CAD build for the part. Positions are in the model's coordinates, mm. A direction names the side the tool comes from. Coordinates: 2 decimals unless noted, no trailing zeros. Order: outer loops, then holes, each group sorted by start corner. A loop starts at its lowest first (then second) coordinate and runs counter-clockwise, first axis right, second up. Notation, with made-up numbers: (-14.75, 54.25) - (9.25, 54.25) arc R16 ccw to (9.25, 83.25) - close; hole circle Ø8 at (82, 89.5). An arc over 180 degrees is marked (long way). Return JSON: item names as keys, results as strings.
from build123d import *

# Parameters (mm, degrees)
EXTRUDE_1_DEPTH                 = 220
SKETCH_3_W                      = 130
SKETCH_3_H                      = 90
CUT_EXTRUDE_1_DEPTH             = 585.29444632
EXTRUDE_5_DEPTH                 = 10
EXTRUDE_START                   = -130
EXTRUDE_6_DEPTH                 = 260
EXTRUDE_START_2                 = -220
EXTRUDE_6_2_DEPTH               = 125
EXTRUDE_START_3                 = 95
EXTRUDE_6_3_DEPTH               = 125
EXTRUDE_START_4                 = -76.923226389
EXTRUDE_6_4_DEPTH               = 136.923226389
CUT_EXTRUDE_2_DEPTH             = 585.29444632
SKETCH_13_W                     = 90
SKETCH_13_H                     = 60
EXTRUDE_7_DEPTH                 = 10
EXTRUDE_10_REACH                = 649.534
SKETCH_16_W                     = 90
SKETCH_16_H                     = 60
EXTRUDE_10_DIRECTION_2_REACH    = 649.534
SKETCH_17_W                     = 65
SKETCH_17_H                     = 190
SKETCH_17_W_2                   = 95
EXTRUDE_15_DEPTH                = 5
CUT_EXTRUDE_3_REACH             = 649.534
CUT_EXTRUDE_3_DIRECTION_2_REACH = 649.534


with BuildPart() as part:
    # Эскиз1 → Бобышка-Вытянуть1 (new, symmetric)
    with BuildSketch(Plane.XY):
        Polygon((-219.125113365, -100), (219.125113365, -100), (530, -45.184369862), (530, -55.33863598), (220, -110), (-220, -110), (-530, -55.33863598), (-530, -45.184369862), align=None)
    extrude(amount=EXTRUDE_1_DEPTH, both=True)

    # Эскиз3 → Вырез-Вытянуть1 (cut, through all)
    with BuildSketch(Plane(origin=(0, 0, 0), x_dir=(1, 0, 0), z_dir=(0, 1, 0))):
        with Locations((-465, 175)):
            Rectangle(SKETCH_3_W, SKETCH_3_H)
        with Locations((465, 175)):
            Rectangle(SKETCH_3_W, SKETCH_3_H)
        with Locations((465, -175)):
            Rectangle(SKETCH_3_W, SKETCH_3_H)
        with Locations((-465, -175)):
            Rectangle(SKETCH_3_W, SKETCH_3_H)
    extrude(amount=-CUT_EXTRUDE_1_DEPTH, mode=Mode.SUBTRACT)

    # Эскиз9 → Бобышка-Вытянуть5 (add)
    with BuildSketch(Plane.XY.offset(130)):
        Polygon((-530, -45.184369862), (-400, -68.106877354), (-400, 60), (-530, 60), align=None)
        Polygon((400, -68.106877354), (400, 60), (530, 60), (530, -45.184369862), align=None)
    extrude_5 = extrude(amount=-EXTRUDE_5_DEPTH)

    # Зеркальное отражение3: Бобышка-Вытянуть5 across plane
    add(extrude_5.mirror(Plane.XY))

    # Бобышка-Вытянуть6: read off the stored shape, not the designer's step
    # Бобышка-Вытянуть6 outline → Бобышка-Вытянуть6 (add)
    with BuildSketch(Plane.XY.offset(EXTRUDE_START)):
        Polygon((-530, 60), (-530, -45.184369862), (-520, -46.947639669), (-520, 60), align=None)
        Polygon((530, -45.184369862), (530, 60), (520, 60), (520, -46.947639669), align=None)
    extrude(amount=EXTRUDE_6_DEPTH)

    # Extrude 6 2 outline → Extrude 6 2 (add)
    with BuildSketch(Plane.XY.offset(EXTRUDE_START_2)):
        Polygon((-350, 60), (-350, -76.923226389), (-340, -78.686496196), (-340, 60), align=None)
        Polygon((350, -76.923226389), (350, 60), (340, 60), (340, -78.686496196), align=None)
    extrude(amount=EXTRUDE_6_2_DEPTH)

    # Extrude 6 3 outline → Extrude 6 3 (add)
    with BuildSketch(Plane.XY.offset(EXTRUDE_START_3)):
        Polygon((-350, 60), (-350, -76.923226389), (-340, -78.686496196), (-340, 60), align=None)
        Polygon((350, -76.923226389), (350, 60), (340, 60), (340, -78.686496196), align=None)
    extrude(amount=EXTRUDE_6_3_DEPTH)

    # Extrude 6 4 outline → Extrude 6 4 (add)
    with BuildSketch(Plane(origin=(0, 0, 0), x_dir=(1, 0, 0), z_dir=(0, 1, 0)).offset(EXTRUDE_START_4)):
        Polygon((350, -105), (385.56624327, -105), (400, -130), (400, -120), (405.773502692, -120), (391.339745962, -95), (350, -95), align=None)
        Polygon((-400, -130), (-385.56624327, -105), (-350, -105), (-350, -95), (-391.339745962, -95), (-405.773502692, -120), (-400, -120), align=None)
        Polygon((-400, 120), (-405.773502692, 120), (-391.339745962, 95), (-350, 95), (-350, 105), (-385.56624327, 105), (-400, 130), align=None)
        Polygon((400, 130), (385.56624327, 105), (350, 105), (350, 95), (391.339745962, 95), (405.773502692, 120), (400, 120), align=None)
    extrude(amount=EXTRUDE_6_4_DEPTH)

    # Эскиз12 → Вырез-Вытянуть2 (cut, through all)
    with BuildSketch(Plane(origin=(0, 0, 0), x_dir=(1, 0, 0), z_dir=(0, 1, 0))):
        Polygon((350, -105), (350, -220), (400, -220), (400, -130), (385.56624327, -105), align=None)
        Polygon((400, 220), (350, 220), (350, 105), (385.56624327, 105), (400, 130), align=None)
        Polygon((-400, -220), (-350, -220), (-350, -105), (-385.56624327, -105), (-400, -130), align=None)
        Polygon((-400, 130), (-385.56624327, 105), (-350, 105), (-350, 220), (-400, 220), align=None)
    extrude(amount=-CUT_EXTRUDE_2_DEPTH, mode=Mode.SUBTRACT)

    # Эскиз13 → Бобышка-Вытянуть7 (add)
    # profile 1 of 2: a face of its own
    with BuildSketch(Plane.XY.offset(220)):
        Polygon((-296.831216351, 185), (-369, 60), (-369, -83.727279874), (-350, -87.077492508), (-350, 60), (-340, 60), (-340, -78.686496196), (-219.125113365, -100), (219.125113365, -100), (340, -78.686496196), (340, 60), (350, 60), (350, -87.077492508), (369, -83.727279874), (369, 60), (296.831216351, 185), (255.81415713, 185), (225, 300), (220, 300), (220, -60), (-220, -60), (-220, 300), (-225, 300), (-255.81415713, 185), align=None)
        with Locations((-274, 90)):
            Rectangle(SKETCH_13_W, SKETCH_13_H, mode=Mode.SUBTRACT)
        with Locations((274, 90)):
            Rectangle(SKETCH_13_W, SKETCH_13_H, mode=Mode.SUBTRACT)
    # profile 2 of 2: a face of its own
    with BuildSketch(Plane.XY.offset(220)):
        Polygon((-350, 60), (-350, -87.077492508), (-220, -110), (220, -110), (350, -87.077492508), (350, 60), (340, 60), (340, -78.686496196), (219.125113365, -100), (-219.125113365, -100), (-340, -78.686496196), (-340, 60), align=None)
    extrude_7 = extrude(amount=-EXTRUDE_7_DEPTH)

    # Зеркальное отражение4: Бобышка-Вытянуть7 across plane
    add(extrude_7.mirror(Plane.XY))

    # Эскиз16 → Бобышка-Вытянуть10 (add, up to next)
    with BuildSketch(Plane.XY, mode=Mode.PRIVATE) as extrude_10_sk1:
        Polygon((369, 60), (296.831216351, 185), (255.81415713, 185), (225, 300), (220, 300), (220, -60), (-220, -60), (-220, 300), (-225, 300), (-255.81415713, 185), (-296.831216351, 185), (-369, 60), (-369, 55), (-359, 55), (-350, 55), (-350, 60), (-357.452994616, 60), (-324, 117.942286341), (-324, 55), (-230, 55), (-230, -70), (230, -70), (230, 55), (324, 55), (324, 117.942286341), (357.452994616, 60), (350, 60), (350, 55), (359, 55), (369, 55), align=None)
        Polygon((-291.057713659, 175), (-248.14088725, 175), (-230, 242.702712911), (-230, 125), (-319.925227119, 125), align=None, mode=Mode.SUBTRACT)
        Polygon((230, 242.702712911), (230, 125), (319.925227119, 125), (291.057713659, 175), (248.14088725, 175), align=None, mode=Mode.SUBTRACT)
        with Locations((-274, 90)):
            Rectangle(SKETCH_16_W, SKETCH_16_H, mode=Mode.SUBTRACT)
        with Locations((274, 90)):
            Rectangle(SKETCH_16_W, SKETCH_16_H, mode=Mode.SUBTRACT)
    extrude_10_tool1 = extrude(extrude_10_sk1.sketch, amount=EXTRUDE_10_REACH, mode=Mode.PRIVATE) - part.part
    add(extrude_10_tool1.solids().sort_by_distance((325.766077, 118.372216, 0))[0])

    # Эскиз16 → Бобышка-Вытянуть10 direction 2 (add, up to next)
    with BuildSketch(Plane.XY, mode=Mode.PRIVATE) as extrude_10_direction_2_sk1:
        Polygon((369, 60), (296.831216351, 185), (255.81415713, 185), (225, 300), (220, 300), (220, -60), (-220, -60), (-220, 300), (-225, 300), (-255.81415713, 185), (-296.831216351, 185), (-369, 60), (-369, 55), (-359, 55), (-350, 55), (-350, 60), (-357.452994616, 60), (-324, 117.942286341), (-324, 55), (-230, 55), (-230, -70), (230, -70), (230, 55), (324, 55), (324, 117.942286341), (357.452994616, 60), (350, 60), (350, 55), (359, 55), (369, 55), align=None)
        Polygon((-291.057713659, 175), (-248.14088725, 175), (-230, 242.702712911), (-230, 125), (-319.925227119, 125), align=None, mode=Mode.SUBTRACT)
        Polygon((230, 242.702712911), (230, 125), (319.925227119, 125), (291.057713659, 175), (248.14088725, 175), align=None, mode=Mode.SUBTRACT)
        with Locations((-274, 90)):
            Rectangle(SKETCH_16_W, SKETCH_16_H, mode=Mode.SUBTRACT)
        with Locations((274, 90)):
            Rectangle(SKETCH_16_W, SKETCH_16_H, mode=Mode.SUBTRACT)
    extrude_10_direction_2_tool1 = extrude(extrude_10_direction_2_sk1.sketch, amount=-EXTRUDE_10_DIRECTION_2_REACH, mode=Mode.PRIVATE) - part.part
    add(extrude_10_direction_2_tool1.solids().sort_by_distance((325.766077, 118.372216, 0))[0])

    # Эскиз17 → Бобышка-Вытянуть15 (add)
    # profile 1 of 2: a face of its own
    with BuildSketch(Plane(origin=(0, 60, 0), x_dir=(1, 0, 0), z_dir=(0, 1, 0))):
        Polygon((-391.339745962, -95), (-369, -95), (-369, 95), (-391.339745962, 95), (-405.773502692, 120), (-520, 120), (-520, -120), (-405.773502692, -120), align=None)
        with Locations((-437.5, 0)):
            Rectangle(SKETCH_17_W, SKETCH_17_H, mode=Mode.SUBTRACT)
    # profile 2 of 2: a face of its own
    with BuildSketch(Plane(origin=(0, 60, 0), x_dir=(1, 0, 0), z_dir=(0, 1, 0))):
        Polygon((385.56624327, 105), (369, 105), (369, -105), (385.56624327, -105), (400, -130), (530, -130), (530, 130), (400, 130), align=None)
        with Locations((452.5, 0)):
            Rectangle(SKETCH_17_W_2, SKETCH_17_H, mode=Mode.SUBTRACT)
    extrude(amount=-EXTRUDE_15_DEPTH)

    # Вырез-Вытянуть3: up to this face of the body (flat: up to its plane)
    cut_extrude_3_end = Plane(part.part.faces().sort_by_distance((-437.5, 57.5, -95))[0])
    # Эскиз18 → Вырез-Вытянуть3 (cut, up to the picked face)
    with BuildSketch(Plane.XY, mode=Mode.PRIVATE) as cut_extrude_3_sk1:
        with BuildLine():
            Line((-405, 55), (-405, 60))
            Line((-405, 60), (-402.5, 60))
            Line((-402.5, 60), (-402.5, 57.5))
            ThreePointArc((-402.5, 57.5), (-403.232233047, 55.732233047), (-405, 55))
        make_face()
    cut_extrude_3_tool1 = split(extrude(cut_extrude_3_sk1.sketch, amount=-CUT_EXTRUDE_3_REACH, mode=Mode.PRIVATE), bisect_by=cut_extrude_3_end, keep=Keep.BOTH, mode=Mode.PRIVATE)
    # Эскиз18 → Вырез-Вытянуть3 (cut, up to the picked face)
    with BuildSketch(Plane.XY, mode=Mode.PRIVATE) as cut_extrude_3_sk2:
        with BuildLine():
            Line((405, 55), (405, 60))
            Line((405, 60), (402.5, 60))
            Line((402.5, 60), (402.5, 57.5))
            ThreePointArc((402.5, 57.5), (403.232233047, 55.732233047), (405, 55))
        make_face()
    cut_extrude_3_tool2 = split(extrude(cut_extrude_3_sk2.sketch, amount=-CUT_EXTRUDE_3_REACH, mode=Mode.PRIVATE), bisect_by=cut_extrude_3_end, keep=Keep.BOTH, mode=Mode.PRIVATE)
    add(cut_extrude_3_tool1.solids().sort_by(Axis((-403.833127, 57.733375, 0), (0, 0, -1)))[0], mode=Mode.SUBTRACT)
    add(cut_extrude_3_tool2.solids().sort_by(Axis((403.833127, 57.733375, 0), (0, 0, -1)))[0], mode=Mode.SUBTRACT)

    # Вырез-Вытянуть3 direction 2: up to this face of the body (flat: up to its plane)
    cut_extrude_3_direction_2_end = Plane(part.part.faces().sort_by_distance((-437.5, 57.5, 95))[0])
    # Эскиз18 → Вырез-Вытянуть3 direction 2 (cut, up to the picked face)
    with BuildSketch(Plane.XY, mode=Mode.PRIVATE) as cut_extrude_3_direction_2_sk1:
        with BuildLine():
            Line((-405, 55), (-405, 60))
            Line((-405, 60), (-402.5, 60))
            Line((-402.5, 60), (-402.5, 57.5))
            ThreePointArc((-402.5, 57.5), (-403.232233047, 55.732233047), (-405, 55))
        make_face()
    cut_extrude_3_direction_2_tool1 = split(extrude(cut_extrude_3_direction_2_sk1.sketch, amount=CUT_EXTRUDE_3_DIRECTION_2_REACH, mode=Mode.PRIVATE), bisect_by=cut_extrude_3_direction_2_end, keep=Keep.BOTH, mode=Mode.PRIVATE)
    # Эскиз18 → Вырез-Вытянуть3 direction 2 (cut, up to the picked face)
    with BuildSketch(Plane.XY, mode=Mode.PRIVATE) as cut_extrude_3_direction_2_sk2:
        with BuildLine():
            Line((405, 55), (405, 60))
            Line((405, 60), (402.5, 60))
            Line((402.5, 60), (402.5, 57.5))
            ThreePointArc((402.5, 57.5), (403.232233047, 55.732233047), (405, 55))
        make_face()
    cut_extrude_3_direction_2_tool2 = split(extrude(cut_extrude_3_direction_2_sk2.sketch, amount=CUT_EXTRUDE_3_DIRECTION_2_REACH, mode=Mode.PRIVATE), bisect_by=cut_extrude_3_direction_2_end, keep=Keep.BOTH, mode=Mode.PRIVATE)
    add(cut_extrude_3_direction_2_tool1.solids().sort_by(Axis((-403.833127, 57.733375, 0), (0, 0, 1)))[0], mode=Mode.SUBTRACT)
    add(cut_extrude_3_direction_2_tool2.solids().sort_by(Axis((403.833127, 57.733375, 0), (0, 0, 1)))[0], mode=Mode.SUBTRACT)


solid = part.part
Item 1: Band-saw the part on C-C, the plane x = -422. List the corners of the cut face in (y, z), then the cut area to 3 significant figures.
Findings below:
{"outline": "(-74.38, -130) - (60, -130) - (60, -95) - (55, -95) - (55, -120) - (-64.23, -120) - (-64.23, 120) - (55, 120) - (55, 95) - (60, 95) - (60, 130) - (-74.38, 130) - close", "area": "5,370 mm²"}
Item 2: Which spindle directions (+Z, -Z, +X, -X, +Y, -Y) get a long thin tool onto all of the face, cutting with end or side? Do faces 4 (the flat face through (229, 90, -3)), 5 (the flat face through (276, 55, -3)), 6 (the flat face through (368, -15, 105)). Say none if no direction does.
Findings below:
{"face 4": "+Z, -Z", "face 5": "none", "face 6": "-Y"}
Item 3: Wall check: L1, parallel to X at y = 46.5, z = -184.5; L2, parallel to X at y = -24.5, z = -38; L3, parallel to Y at x = 29, z = -118.5. Give the ranges that are in metal, low to high. Write a range as [from, to].
Findings below:
{"L1": "x = [-350, -340], [-230, -220], [220, 230], [340, 350]", "L2": "x = [-530, -520], [-230, -220], [220, 230], [520, 530]", "L3": "y = [-110, -100], [-70, -60]"}
Item 4: Drop flat-ended pins along their axis: P1, Ø1.5, axis at y = 210.5, z = 132, coming from the -X side; P2, Ø1.5, axis at x = -390, y = 36.5, coming from the +Z side; P3, Ø1, axis at x = -414.5, z = 68, coming from the +Y side. Give the stop position or say it passes through.
Findings below:
{"P1": "stops at x = -249.18", "P2": "stops at z = 113.98", "P3": "stops at y = -65.46"}
Item 5: Band-saw the part on B-B, the plane z = 76. Count the separate pieces of the cut face and the enclosed holes in it, then the cut area to 3 significant figures.
Findings below:
{"separate pieces": "2", "enclosed holes": "4", "area": "33,000 mm²"}
Item 6: Band-saw the part on A-A, the plane x = -78. List the corners of the cut face in (y, z).
Findings below:
{"outline": "(-110, -220) - (-60, -220) - (-60, 220) - (-110, 220) - close; hole (-100, -210) - (-70, -210) - (-70, 210) - (-100, 210) - close"}
Item 7: Mould opens along Y. For faces 1 (the flat face through (350, -15, -158)), 2 (the flat face through (319, 90, -3)), 3 (the flat face through (240.62, 241.7, 3.08)) say: released by +Y, released by -Y, zero draft, split by the parting line, or undercut.
Findings below:
{"face 1": "zero draft", "face 2": "undercut", "face 3": "released by +Y"}
